```python
from build123d import *

# Parameters (mm, degrees)
BOSS_EXTRUDE1_DEPTH      = 150
BOSS_EXTRUDE1_DEPTH_BACK = 150
SKETCH1_W                = 30
SKETCH1_H                = 60
SKETCH2_R                = 2.5
CUT_EXTRUDE1_DEPTH       = 3
SKETCH3_R                = 4
CUT_EXTRUDE2_DEPTH       = 156.884572681


with BuildPart() as part:
    # Sketch1 → Boss-Extrude1 (new, two sides: drawn at the far end of the back side and taken through both)
    with BuildSketch(Plane.XY.offset(-BOSS_EXTRUDE1_DEPTH_BACK)):
        Rectangle(SKETCH1_W, SKETCH1_H)
    extrude(amount=BOSS_EXTRUDE1_DEPTH + BOSS_EXTRUDE1_DEPTH_BACK)

    # Sketch2 → Cut-Extrude1 (cut)
    with BuildSketch(Plane(origin=(15, 0, 0), x_dir=(0, 0, -1), z_dir=(1, 0, 0))):
        with Locations((0, 18.25)):
            Circle(SKETCH2_R)
        with Locations(Location((0, -18.25, 0), (0, 0, 180))):
            Circle(SKETCH2_R)
    extrude(amount=-CUT_EXTRUDE1_DEPTH, mode=Mode.SUBTRACT)

    # Sketch3 → Cut-Extrude2 (cut, through all)
    with BuildSketch(Plane(origin=(15, 0, 0), x_dir=(0, 0, -1), z_dir=(1, 0, 0))):
        Circle(SKETCH3_R)
    extrude(amount=-CUT_EXTRUDE2_DEPTH, mode=Mode.SUBTRACT)


solid = part.part
```
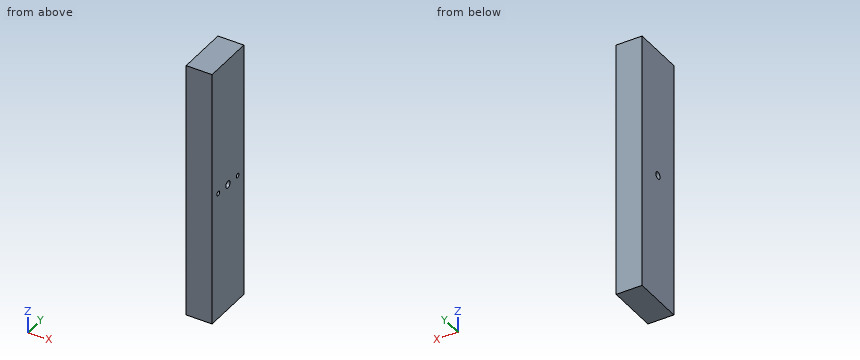
Check sheet for the modelled part. Datum: model origin and axes. Units: mm. Round coordinates to 2 decimals unless told otherwise and drop trailing zeros. Order: outer loops, then holes, each group sorted by start corner. A loop starts at its lowest first (then second) coordinate and runs counter-clockwise, first axis right, second up. Notation, with made-up numbers: (-25, -6) -> (-2, -6) arc R14 ccw to (-2, 15) -> close; hole circle Ø9 at (-9, -5). An arc over 180 degrees is marked (long way). Use CSV: the item, a comma, the result in double quotes.
(1) Cross-section at A-A (y = 0). Record the boundary of the cut face in (x, z).
Worked out:
outline,"(-15, -150) -> (15, -150) -> (15, -4) -> (-15, -4) -> close; (-15, 4) -> (15, 4) -> (15, 150) -> (-15, 150) -> close"
(2) Material ranges on line 1 along Y through (x, z) = (13.5, 0); line 2 along Y through (x, z) = (-5.5, 0); line 3 along Z through (x, y) = (7, -2.5), recorded low to high. Write a range as from..to.
Worked out:
line 1,"-30..-20.75, -15.75..-4, 4..15.75, 20.75..30"
line 2,"-30..-4, 4..30"
line 3,"-150..-3.12, 3.12..150"
(3) Depth check by flat-ended pin: pin 1 (5.5 mm diameter, centred on y = 19, z = -1, fed in from +X). Enter the tip coordinate at first touch or a pass-through.
Worked out:
pin 1,"x = 15"
(4) Cross-section at B-B (z = 0). Record the boundary of the cut face in (x, y), and give its area (3 significant figures).
Worked out:
outline,"(-15, -30) -> (15, -30) -> (15, -20.75) -> (12, -20.75) -> (12, -15.75) -> (15, -15.75) -> (15, -4) -> (-15, -4) -> close; (-15, 4) -> (15, 4) -> (15, 15.75) -> (12, 15.75) -> (12, 20.75) -> (15, 20.75) -> (15, 30) -> (-15, 30) -> close"
area,"1,530 mm²"
